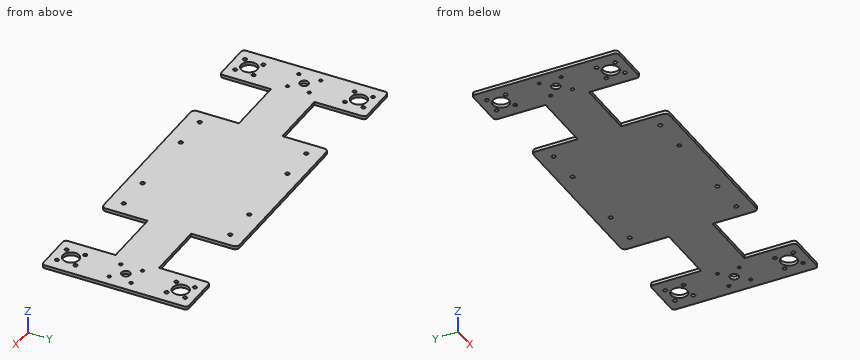
from build123d import *

# Parameters (mm, degrees)
SKETCH_1_R      = 1.5
SKETCH_1_W      = 272.3
SKETCH_1_H      = 40
EXTRUDE_1_DEPTH = 3
FILLET_1_R      = 7
SKETCH_2_W      = 13.425
SKETCH_2_H      = 40
SKETCH_2_W_2    = 33.15
SKETCH_2_W_3    = 66.85
EXTRUDE_2_DEPTH = 3
FILLET_2_R      = 4
SKETCH_3_R      = 1.75
SKETCH_3_R_2    = 7.5
EXTRUDE_3_DEPTH = 3
FILLET_3_R      = 3
FILLET_5_R      = 3


with BuildPart() as part:
    # 스케치1 → 보스-돌출1 (new body)
    # profile 1 of 5: a face of its own
    with BuildSketch(Plane.XY):
        with BuildLine():
            Line((156.15, -4), (156.15, -20))
            Line((156.15, -20), (176.15, -20))
            Line((176.15, -20), (176.15, 20))
            Line((176.15, 20), (156.15, 20))
            Line((156.15, 20), (156.15, 4))
            ThreePointArc((156.15, 4), (158.978427125, 2.828427125), (160.15, 0))
            ThreePointArc((160.15, 0), (158.978427125, -2.828427125), (156.15, -4))
        make_face()
        with Locations((166.15, -10)):
            Circle(SKETCH_1_R, mode=Mode.SUBTRACT)
        with Locations((166.15, 10)):
            Circle(SKETCH_1_R, mode=Mode.SUBTRACT)
    # profile 2 of 5: a face of its own
    with BuildSketch(Plane.XY):
        with BuildLine():
            Line((136.15, 20), (136.15, -20))
            Line((136.15, -20), (156.15, -20))
            Line((156.15, -20), (156.15, -4))
            ThreePointArc((156.15, -4), (152.15, 0), (156.15, 4))
            Line((156.15, 4), (156.15, 20))
            Line((156.15, 20), (136.15, 20))
        make_face()
        with Locations((146.15, -10)):
            Circle(SKETCH_1_R, mode=Mode.SUBTRACT)
        with Locations((146.15, 10)):
            Circle(SKETCH_1_R, mode=Mode.SUBTRACT)
    # profile 3 of 5: a face of its own
    with BuildSketch(Plane.XY):
        Rectangle(SKETCH_1_W, SKETCH_1_H)
    # profile 4 of 5: a face of its own
    with BuildSketch(Plane.XY):
        with BuildLine():
            Line((-176.15, -20), (-156.15, -20))
            Line((-156.15, -20), (-156.15, -4))
            ThreePointArc((-156.15, -4), (-160.15, 0), (-156.15, 4))
            Line((-156.15, 4), (-156.15, 20))
            Line((-156.15, 20), (-176.15, 20))
            Line((-176.15, 20), (-176.15, -20))
        make_face()
        with Locations((-166.15, -10)):
            Circle(SKETCH_1_R, mode=Mode.SUBTRACT)
        with Locations((-166.15, 10)):
            Circle(SKETCH_1_R, mode=Mode.SUBTRACT)
    # profile 5 of 5: a face of its own
    with BuildSketch(Plane.XY):
        with BuildLine():
            Line((-156.15, -4), (-156.15, -20))
            Line((-156.15, -20), (-136.15, -20))
            Line((-136.15, -20), (-136.15, 20))
            Line((-136.15, 20), (-156.15, 20))
            Line((-156.15, 20), (-156.15, 4))
            ThreePointArc((-156.15, 4), (-153.321572875, 2.828427125), (-152.15, 0))
            ThreePointArc((-152.15, 0), (-153.321572875, -2.828427125), (-156.15, -4))
        make_face()
        with Locations((-146.15, -10)):
            Circle(SKETCH_1_R, mode=Mode.SUBTRACT)
        with Locations((-146.15, 10)):
            Circle(SKETCH_1_R, mode=Mode.SUBTRACT)
    extrude(amount=EXTRUDE_1_DEPTH)

    # 필렛1
    fillet_1_edges = [part.edges().sort_by_distance(p)[0] for p in [
        (176.15, 20, 1.5),
        (176.15, -20, 1.5),
        (-176.15, -20, 1.5),
        (-176.15, 20, 1.5),
    ]]
    fillet(fillet_1_edges, radius=FILLET_1_R)

    # 스케치2 → 보스-돌출2 (add)
    with BuildSketch(Plane.XY.offset(3)):
        with BuildLine():
            Line((-80, 62.43), (-80, 20))
            Line((-80, 20), (-66.575, 20))
            Line((-66.575, 20), (-66.575, 47.2))
            ThreePointArc((-66.575, 47.2), (-67.847792206, 50.272792206), (-64.775, 49))
            Line((-64.775, 49), (-35.225, 49))
            ThreePointArc((-35.225, 49), (-33.425, 50.8), (-31.625, 49))
            Line((-31.625, 49), (31.625, 49))
            ThreePointArc((31.625, 49), (33.425, 50.8), (35.225, 49))
            Line((35.225, 49), (64.775, 49))
            ThreePointArc((64.775, 49), (66.575, 50.8), (68.375, 49))
            ThreePointArc((68.375, 49), (67.847792206, 47.727207794), (66.575, 47.2))
            Line((66.575, 47.2), (66.575, 20))
            Line((66.575, 20), (80, 20))
            Line((80, 20), (80, 62.43))
            Line((80, 62.43), (-80, 62.43))
        make_face()
        with Locations((-73.2875, 0)):
            Rectangle(SKETCH_2_W, SKETCH_2_H)
        with BuildLine():
            Line((-80, -20), (-80, -62.43))
            Line((-80, -62.43), (80, -62.43))
            Line((80, -62.43), (80, -20))
            Line((80, -20), (66.575, -20))
            Line((66.575, -20), (66.575, -47.2))
            ThreePointArc((66.575, -47.2), (67.847792206, -47.727207794), (68.375, -49))
            ThreePointArc((68.375, -49), (66.575, -50.8), (64.775, -49))
            Line((64.775, -49), (35.225, -49))
            ThreePointArc((35.225, -49), (33.425, -50.8), (31.625, -49))
            Line((31.625, -49), (-31.625, -49))
            ThreePointArc((-31.625, -49), (-33.425, -50.8), (-35.225, -49))
            Line((-35.225, -49), (-64.775, -49))
            ThreePointArc((-64.775, -49), (-67.847792206, -50.272792206), (-66.575, -47.2))
            Line((-66.575, -47.2), (-66.575, -20))
            Line((-66.575, -20), (-80, -20))
        make_face()
        with Locations((-50, 0)):
            Rectangle(SKETCH_2_W_2, SKETCH_2_H)
        with BuildLine():
            Line((-66.575, 47.2), (-66.575, 20))
            Line((-66.575, 20), (-33.425, 20))
            Line((-33.425, 20), (-33.425, 47.2))
            ThreePointArc((-33.425, 47.2), (-34.697792206, 47.727207794), (-35.225, 49))
            Line((-35.225, 49), (-64.775, 49))
            ThreePointArc((-64.775, 49), (-65.302207794, 47.727207794), (-66.575, 47.2))
        make_face()
        with BuildLine():
            Line((-33.425, 47.2), (-33.425, 20))
            Line((-33.425, 20), (33.425, 20))
            Line((33.425, 20), (33.425, 47.2))
            ThreePointArc((33.425, 47.2), (32.152207794, 47.727207794), (31.625, 49))
            Line((31.625, 49), (-31.625, 49))
            ThreePointArc((-31.625, 49), (-32.152207794, 47.727207794), (-33.425, 47.2))
        make_face()
        Rectangle(SKETCH_2_W_3, SKETCH_2_H)
        with Locations((50, 0)):
            Rectangle(SKETCH_2_W_2, SKETCH_2_H)
        with BuildLine():
            Line((33.425, 20), (66.575, 20))
            Line((66.575, 20), (66.575, 47.2))
            ThreePointArc((66.575, 47.2), (65.302207794, 47.727207794), (64.775, 49))
            Line((64.775, 49), (35.225, 49))
            ThreePointArc((35.225, 49), (34.697792206, 47.727207794), (33.425, 47.2))
            Line((33.425, 47.2), (33.425, 20))
        make_face()
        with BuildLine():
            Line((66.575, -47.2), (66.575, -20))
            Line((66.575, -20), (33.425, -20))
            Line((33.425, -20), (33.425, -47.2))
            ThreePointArc((33.425, -47.2), (34.697792206, -47.727207794), (35.225, -49))
            Line((35.225, -49), (64.775, -49))
            ThreePointArc((64.775, -49), (65.302207794, -47.727207794), (66.575, -47.2))
        make_face()
        with BuildLine():
            Line((-33.425, -20), (-66.575, -20))
            Line((-66.575, -20), (-66.575, -47.2))
            ThreePointArc((-66.575, -47.2), (-65.302207794, -47.727207794), (-64.775, -49))
            Line((-64.775, -49), (-35.225, -49))
            ThreePointArc((-35.225, -49), (-34.697792206, -47.727207794), (-33.425, -47.2))
            Line((-33.425, -47.2), (-33.425, -20))
        make_face()
        with BuildLine():
            Line((33.425, -20), (-33.425, -20))
            Line((-33.425, -20), (-33.425, -47.2))
            ThreePointArc((-33.425, -47.2), (-32.152207794, -47.727207794), (-31.625, -49))
            Line((-31.625, -49), (31.625, -49))
            ThreePointArc((31.625, -49), (32.152207794, -47.727207794), (33.425, -47.2))
            Line((33.425, -47.2), (33.425, -20))
        make_face()
    extrude(amount=-EXTRUDE_2_DEPTH)

    # 필렛2
    fillet_2_edges = [part.edges().sort_by_distance(p)[0] for p in [
        (80, -62.43, 1.5),
        (-80, -62.43, 1.5),
        (-80, 62.43, 1.5),
        (80, 62.43, 1.5),
    ]]
    fillet(fillet_2_edges, radius=FILLET_2_R)

    # 스케치3 → 보스-돌출3 (add)
    # profile 1 of 2: a face of its own
    with BuildSketch(Plane.XY.offset(3)):
        with BuildLine():
            Line((-176.15, -13), (-176.15, -66.970562748))
            Line((-176.15, -66.970562748), (-136.15, -66.970562748))
            Line((-136.15, -66.970562748), (-136.15, -20))
            Line((-136.15, -20), (-169.15, -20))
            ThreePointArc((-169.15, -20), (-174.099747468, -17.949747468), (-176.15, -13))
        make_face()
        with Locations((-164.635281374, -42)):
            Circle(SKETCH_3_R, mode=Mode.SUBTRACT)
        with Locations((-147.664718626, -42)):
            Circle(SKETCH_3_R, mode=Mode.SUBTRACT)
        with Locations((-147.664718626, -58.970562748)):
            Circle(SKETCH_3_R, mode=Mode.SUBTRACT)
        with Locations((-164.635281374, -58.970562748)):
            Circle(SKETCH_3_R, mode=Mode.SUBTRACT)
        with Locations((-156.15, -50.485281374)):
            Circle(SKETCH_3_R_2, mode=Mode.SUBTRACT)
    # profile 2 of 2: a face of its own
    with BuildSketch(Plane.XY.offset(3)):
        with BuildLine():
            Line((-176.15, 66.970562748), (-176.15, 13))
            ThreePointArc((-176.15, 13), (-174.099747468, 17.949747468), (-169.15, 20))
            Line((-169.15, 20), (-136.15, 20))
            Line((-136.15, 20), (-136.15, 66.970562748))
            Line((-136.15, 66.970562748), (-176.15, 66.970562748))
        make_face()
        with Locations((-164.635281374, 42)):
            Circle(SKETCH_3_R, mode=Mode.SUBTRACT)
        with Locations((-147.664718626, 42)):
            Circle(SKETCH_3_R, mode=Mode.SUBTRACT)
        with Locations((-156.15, 50.485281374)):
            Circle(SKETCH_3_R_2, mode=Mode.SUBTRACT)
        with Locations((-164.635281374, 58.970562748)):
            Circle(SKETCH_3_R, mode=Mode.SUBTRACT)
        with Locations((-147.664718626, 58.970562748)):
            Circle(SKETCH_3_R, mode=Mode.SUBTRACT)
    extrude_3 = extrude(amount=-EXTRUDE_3_DEPTH)

    # 필렛3
    fillet_3_edges = [part.edges().sort_by_distance(p)[0] for p in [
        (-176.15, 66.970562748, 1.5),
        (-136.15, 66.970562748, 1.5),
        (-136.15, -66.970562748, 1.5),
        (-176.15, -66.970562748, 1.5),
    ]]
    fillet(fillet_3_edges, radius=FILLET_3_R)

    # 대칭 복사1: 보스-돌출3 across plane
    add(extrude_3.mirror(Plane(origin=(0, 0, 0), x_dir=(0, 0, 1), z_dir=(1, 0, 0))))

    # 필렛5
    fillet_5_edges = [part.edges().sort_by_distance(p)[0] for p in [
        (136.15, 66.970562748, 1.5),
        (176.15, 66.970562748, 1.5),
        (176.15, -66.970562748, 1.5),
        (136.15, -66.970562748, 1.5),
    ]]
    fillet(fillet_5_edges, radius=FILLET_5_R)


solid = part.part
The listing builds one solid part. Answer for the finished solid, in the listing's coordinates (mm). Coordinates: 2 decimals unless noted, no trailing zeros. Loops run counter-clockwise (first coordinate to the right, second up) from the corner with the lowest first, then second, coordinate; pieces in that order, holes last.
1) Find section D-D on x = 107.5. Write down the section's boundary in (y, z).
2) Find section B-B on x = 59. Write down the section's boundary in (y, z), then the cut area to 3 significant figures.
3) Flat-ended cylindrical pins translate along their axes: pin 1 Ø5.5 at (x, y) = (147.66, 58.97) entering from +Z; pin 2 Ø2.5 at (x, y) = (-146.15, -10) entering from +Z; pin 3 Ø0.9 at (x, z) = (25.5, 1.5) entering from -Y. Find the tip coordinate at first contact, or state that the pin passes through.
4) Find section A-A on y = 37. Write down the section's boundary in (x, z), then the cut area to 3 significant figures.
5) Find the intervals of material crossed by L1, parallel to X at y = -32.5, z = 0.6; L2, parallel to Y at x = -33, z = 0.5; L3, parallel to X at y = 0.5, z = 1, in increasing order.
6) Find section C-C on z = 1.2. Give the number of separate pieces and of enclosed holes in the cut face, then the cut area to 3 significant figures.
Values:
1. outline: (-20, 0) - (20, 0) - (20, 3) - (-20, 3) - close
2. outline: (-62.43, 0) - (62.43, 0) - (62.43, 3) - (-62.43, 3) - close
2. area: 375 mm2
3. pin 1: stops at z = 3
3. pin 2: passes through
3. pin 3: stops at y = -62.43
4. outline: (-176.15, 0) - (-136.15, 0) - (-136.15, 3) - (-176.15, 3) - close; (-80, 0) - (80, 0) - (80, 3) - (-80, 3) - close; (136.15, 0) - (176.15, 0) - (176.15, 3) - (136.15, 3) - close
4. area: 720 mm2
5. L1: x = -176.15 to -136.15, -80 to 80, 136.15 to 176.15
5. L2: y = -62.43 to -50.75, -47.25 to 47.25, 50.75 to 62.43
5. L3: x = -176.15 to -160.12, -152.18 to 152.18, 160.12 to 176.15
6. separate pieces: 1
6. enclosed holes: 38
6. area: 34,100 mm2
